from build123d import *

# Parameters (mm, degrees)
FILLET1_R    = 0.4
RECPAT_COUNT = 2
RECPAT_ANGLE = 90


with BuildPart() as part:
    # BodySke → Base-Revolve (revolve)
    with BuildSketch(Plane.XY, mode=Mode.PRIVATE) as base_revolve_sk:
        with BuildLine():
            Line((4.8, 4), (4.8, 8.2))
            Line((4.8, 8.2), (4.79, 8.2))
            Line((4.79, 8.2), (1.7, 7.92966003))
            ThreePointArc((1.7, 7.92966003), (0.429774249, 4.054920104), (0, 0))
            Line((0, 0), (39.8, 0))
            Line((39.8, 0), (39.8, 4))
            Line((39.8, 4), (4.8, 4))
        make_face()
    revolve(base_revolve_sk.sketch.rotate(Axis((1.7, 0, 0), (1, 0, 0)), 90), axis=Axis((1.7, 0, 0), (1, 0, 0)))

    # Fillet1
    fillet1_edges = [part.edges().sort_by_distance(p)[0] for p in [
        (4.8, 0, -4),
    ]]
    fillet(fillet1_edges, radius=FILLET1_R)

    # Sketch3 → Recess section 0
    with BuildSketch(Plane(origin=(0, 0, 0), x_dir=(0, 0, -1), z_dir=(1, 0, 0))):
        with BuildLine():
            Line((0.71, -3.9), (-0.71, -3.9))
            Line((-0.71, -3.9), (-0.71, 3.9))
            Line((-0.71, 3.9), (0.71, 3.9))
            Line((0.71, 3.9), (0.71, -3.9))
        make_face()
    # Sketch4 → Recess section 1
    with BuildSketch(Plane(origin=(4.36, 0, 0), x_dir=(0, 0, -1), z_dir=(1, 0, 0))):
        with BuildLine():
            Line((0.71, -1.726184552), (-0.71, -1.726184552))
            Line((-0.71, -1.726184552), (-0.71, 1.726184552))
            Line((-0.71, 1.726184552), (0.71, 1.726184552))
            Line((0.71, 1.726184552), (0.71, -1.726184552))
        make_face()
    recess = loft(mode=Mode.SUBTRACT)

    # RecPat: Recess ×2 about axis
    recpat_axis = Axis((0, 0, 0), (1, 0, 0))
    for i in range(1, RECPAT_COUNT):
        add(recess.rotate(recpat_axis, i * RECPAT_ANGLE / (RECPAT_COUNT - 1)), mode=Mode.SUBTRACT)

    # RecCorSke → RecessCore (revolve, cut)
    with BuildSketch(Plane.XY, mode=Mode.PRIVATE) as recesscore_sk:
        Polygon((0, 0), (0, 1.5853809), (4.36, 1.2805), (4.776059671, 0), align=None)
    revolve(recesscore_sk.sketch.rotate(Axis((-3.175, 0, 0), (1, 0, 0)), 10.822716804), axis=Axis((-3.175, 0, 0), (1, 0, 0)), mode=Mode.SUBTRACT)


solid = part.part
The model under review builds one solid part; all positions refer to its coordinate system, in mm. A direction names the side the tool comes from. Give positions to 0.01 mm unless a question says otherwise; leave off trailing zeros. Loops run counter-clockwise (first coordinate to the right, second up) from the corner with the lowest first, then second, coordinate; pieces in that order, holes last. Notation, with made-up numbers: (-23.75, 62.25) -> (-5.75, 62.25) arc R14 ccw to (-5.75, 67.25) -> close; hole circle Ø5 at (7.25, 13). An arc over 180 degrees is marked (long way). Write each question's results on one line, items separated by ' | '.
1) Take a section at A-A, the plane x = 36. Give the boundary of the cut face in (y, z), plus the area to 3 significant figures.
Conclusion:
outline: circle Ø8 at (0, 0) | area: 50.3 mm^2
2) Draft analysis for pull direction Y (two halves, no side actions). For faces 1 (the face through (39.8, 0, 0)), 2 (the face through (2.39, 2.71, 0.01)), 3 (the face through (2.537, -7.935, -1.042)), state which applies: pulls with the +Y half, pulls with the -Y half, needs draft (parallel to the pull), parting line crosses it, or undercut.
Conclusion:
face 1: needs draft | face 2: undercut | face 3: parting line crosses it
3) Insertion check: pin 1 Ø2 at (y, z) = (5.5, -4.5) entering from +X; pin 2 Ø4 at (x, y) = (22, -4.5) entering from -Z; pin 3 Ø5 at (x, y) = (13, -2.5) entering from +Z. Each pin has a flat end and moves straight along its axis. Give the tip position at first contact, or say it passes through.
Conclusion:
pin 1: stops at x = 4.8 | pin 2: stops at z = -3.12 | pin 3: stops at z = 4
4) Tool access review of faces 4 (the face through (2.39, -2.71, -0.01)), 5 (the face through (22.258, 3.905, -0.867)): name each direction out of +Z, -Z, +X, -X, +Y, -Y from which nothing blocks a thin tool from reaching the whole face with its end or side.
Conclusion:
face 4: -X | face 5: +X
5) For line 1 along X through (y, z) = (-3.25, -1.75); line 2 along X through (y, z) = (-6.5, -4.5); line 3 along Z through (x, y) = (28, 1.5), list the stretches that pass through material, from the lowest coordinate up. Write a range as from..to.
Conclusion:
line 1: x = 0.36..39.8 | line 2: x = 1.69..4.8 | line 3: z = -3.71..3.71
